```python
from build123d import *


with BuildPart() as part:
    # Schizzo1 → Rivoluzione1 (revolve)
    with BuildSketch(Plane(origin=(0, 0, 0), x_dir=(1, 0, 0), z_dir=(0, 1, 0)), mode=Mode.PRIVATE) as rivoluzione1_sk:
        with BuildLine():
            Line((0, 3.9), (0, 6.1))
            Line((0, 6.1), (21.7, 6.1))
            ThreePointArc((21.7, 6.1), (21.841421356, 6.158578644), (21.9, 6.3))
            Line((21.9, 6.3), (21.9, 8))
            Line((21.9, 8), (25.2, 8))
            Line((25.2, 8), (25.2, 3.9))
            Line((25.2, 3.9), (0, 3.9))
        make_face()
    revolve(rivoluzione1_sk.sketch.rotate(Axis((-60.499740909, 0, 0), (1, 0, 0)), 180), axis=Axis((-60.499740909, 0, 0), (1, 0, 0)))


solid = part.part
```
Input: part model. Units: mm. Frame: model coordinates. A direction names the side the tool comes from. Give positions to 0.01 mm unless a question says otherwise; leave off trailing zeros. Order: outer loops, then holes, each group sorted by start corner. A loop starts at its lowest first (then second) coordinate and runs counter-clockwise, first axis right, second up. Notation, with made-up numbers: (45.25, 83) - (59.25, 83) arc R26 cw to (59.25, 121) - close; hole circle Ø9 at (-26, 26). An arc over 180 degrees is marked (long way). Use a Markdown table: item, result.
(1) Access query for faces 1 (the flat face through (25.2, -4, 2)), 2 (the flat face through (21.9, 6.5, 0)). Directions: +Z, -Z, +X, -X, +Y, -Y. A direction counts if a zero-diameter tool reaches every point of the face in a straight line with its end or side. Return the directions, or none.
Computed values:
| item | result |
|---|---|
| face 1 | +Z, -Z, +X, +Y, -Y |
| face 2 | -X |
(2) Section query A-A (z = 0). Output: boundary loops of the cut face in (x, y).
Computed values:
| item | result |
|---|---|
| outline | (0, -6.1) - (21.7, -6.1) arc R0.2 cw to (21.9, -6.3) - (21.9, -8) - (25.2, -8) - (25.2, -3.9) - (0, -3.9) - close; (0, 3.9) - (25.2, 3.9) - (25.2, 8) - (21.9, 8) - (21.9, 6.3) arc R0.2 cw to (21.7, 6.1) - (0, 6.1) - close |
(3) Pin query (flat end, axial travel): pin 1 (2 mm diameter, centred on x = 8.5, y = -6, fed in from -Z); pin 2 (6 mm diameter, centred on x = 16, z = -3.5, fed in from +Y); pin 3 (6 mm diameter, centred on x = 22, z = -3.5, fed in from +Y). Return the tip coordinate at first contact, or that it passes through.
Computed values:
| item | result |
|---|---|
| pin 1 | stops at z = -3.49 |
| pin 2 | stops at y = 6.08 |
| pin 3 | stops at y = 7.98 |
(4) Section query C-C (x = 2). Output: boundary loops of the cut face in (y, z).
Computed values:
| item | result |
|---|---|
| outline | circle Ø12.2 at (0, 0); hole circle Ø7.8 at (0, 0) |
(5) Line query: line 1 (Y direction, x = 12.25, z = 0); line 2 (Y direction, x = 22.5, z = 0); line 3 (Z direction, x = 15.5, y = -0.5). Output: solid intervals per line, ascending. Write a range as from..to.
Computed values:
| item | result |
|---|---|
| line 1 | y = -6.1..-3.9, 3.9..6.1 |
| line 2 | y = -8..-3.9, 3.9..8 |
| line 3 | z = -6.08..-3.87, 3.87..6.08 |
(6) Draft query along Z for faces 3 (the flat face through (0, 1, -4)), 4 (the cylindrical face through (11.002, -0.268, -6.094)), 5 (the cylindrical face through (12.42, -2.64, -2.87)). Return one class per face: released by +Z, released by -Z, zero draft, split by the parting line, or undercut.
Computed values:
| item | result |
|---|---|
| face 3 | zero draft |
| face 4 | split by the parting line |
| face 5 | undercut |
(7) Section query D-D (y = -7). Output: boundary loops of the cut face in (x, z), then the cut area to 3 significant figures.
Computed values:
| item | result |
|---|---|
| outline | (21.9, -3.87) - (25.2, -3.87) - (25.2, 3.87) - (21.9, 3.87) - close |
| area | 25.6 mm2 |
